Design review of the part built by this model. Coordinates are the model's own, in mm. Give positions to 0.01 mm unless a question says otherwise; leave off trailing zeros. Order: outer loops, then holes, each group sorted by start corner. A loop starts at its lowest first (then second) coordinate and runs counter-clockwise, first axis right, second up. Notation, with made-up numbers: (59.25, 55.25) -> (72.25, 55.25) arc R31 cw to (72.25, 90.25) -> close; hole circle Ø4 at (18.5, 56). An arc over 180 degrees is marked (long way). One line per item, written item: value. Start each with the question number.
1) Consider section B-B (z = 34.25). State the section outline as (x, y) points.
2) Consider section A-A (x = -27.5). State the section outline as (y, z) points, plus the area to 3 significant figures.
3) For pin 1 (1 mm diameter, centred on x = -35.5, y = -6, fed in from -Z); pin 2 (3 mm diameter, centred on x = -22, y = -5, fed in from +Z), all flat-tipped, find the tip position at first contact; note any pin that passes through.
4) Wall thickness on line 1 along Y through (x, z) = (-24, 37.5); line 2 along Z through (x, y) = (-44, -3.5); line 3 along X through (y, z) = (-4, 37): over which ranges is each line inside the solid? List them lowest first. Write a range as from..to.
from build123d import *

# Parameters (mm, degrees)
F1_DEPTH = 7.112
F2_R     = 3.81


with BuildPart() as f1:
    # F0 (on Front) → F1 (new body)
    with BuildSketch(Plane.XZ):
        with BuildLine():
            Line((-19.773078, 41.113582), (-53.155455, 41.113582))
            ThreePointArc((-53.155455, 41.113582), (-57.645583, 39.25371), (-59.505455, 34.763582))
            Line((-59.505455, 34.763582), (-59.505455, 29.029039))
            ThreePointArc((-59.505455, 29.029039), (-57.645583, 24.53891), (-53.155455, 22.679039))
            Line((-53.155455, 22.679039), (-19.773078, 22.679039))
            ThreePointArc((-19.773078, 22.679039), (-15.28295, 24.53891), (-13.423078, 29.029039))
            Line((-13.423078, 29.029039), (-13.423078, 34.763582))
            ThreePointArc((-13.423078, 34.763582), (-15.28295, 39.25371), (-19.773078, 41.113582))
        make_face()
    extrude(amount=F1_DEPTH)

    # F2
    f2_edges = [f1.edges().sort_by_distance(p)[0] for p in [
        (-13.423078, -7.112, 31.89631),
        (-15.28295, -7.112, 39.25371),
        (-36.464266, -7.112, 41.113582),
        (-57.645583, -7.112, 39.25371),
        (-59.505455, -7.112, 31.89631),
        (-57.645583, -7.112, 24.53891),
        (-36.464266, -7.112, 22.679039),
        (-15.28295, -7.112, 24.53891),
    ]]
    fillet(f2_edges, radius=F2_R)


solid = f1.part
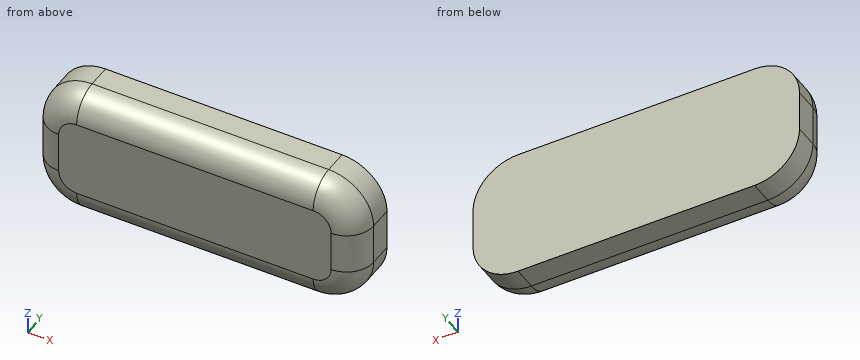
Checked values:
1. outline: (-59.51, -3.3) arc R3.81 ccw to (-55.7, -7.11) -> (-17.23, -7.11) arc R3.81 ccw to (-13.42, -3.3) -> (-13.42, 0) -> (-59.51, 0) -> close
2. outline: (-7.11, 26.49) arc R3.81 ccw to (-3.3, 22.68) -> (0, 22.68) -> (0, 41.11) -> (-3.3, 41.11) arc R3.81 ccw to (-7.11, 37.3) -> close
2. area: 125 mm^2
3. pin 1: stops at z = 23.38
3. pin 2: stops at z = 41.11
4. line 1: y = -7.11..0
4. line 2: z = 22.68..41.11
4. line 3: x = -59.03..-13.9
